Geometry check sheet. Reference: drawing and pictorial views, mm from the part's lowest x, y, z. Coordinates: 2 decimals unless noted, no trailing zeros. Loops run counter-clockwise (first coordinate to the right, second up) from the corner with the lowest first, then second, coordinate; pieces in that order, holes last. Notation, with made-up numbers: (75.5, -27) -> (80.5, -27) arc R30 cw to (80.5, -4) -> close; hole circle Ø8 at (83, 40). An arc over 180 degrees is marked (long way). Answer as a JSON object with one key per item and string values.
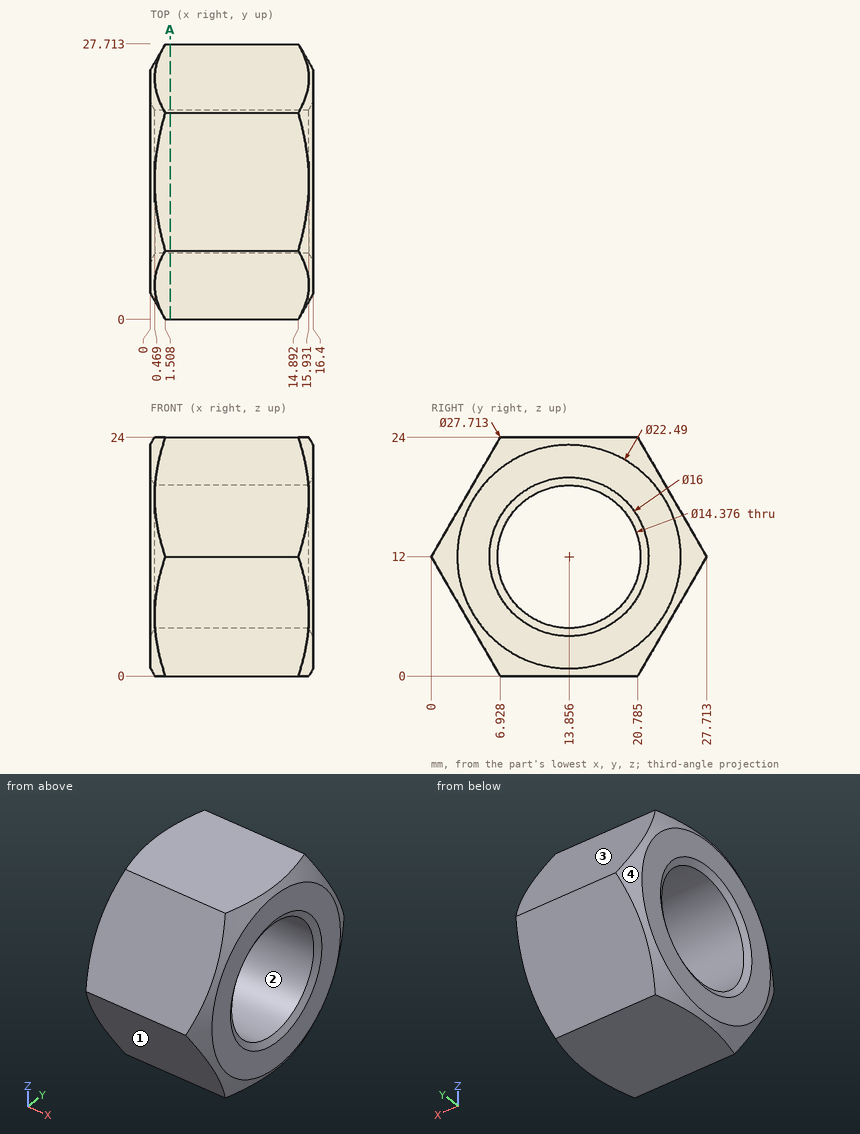
1. Section check A-A, the plane x = 2. Record the boundary of the cut face in (y, z) (1 decimal).
Evaluation:
{"outline": "(0, 12) -> (6.9, 0) -> (20.8, 0) -> (27.7, 12) -> (20.8, 24) -> (6.9, 24) -> close; hole circle Ø14.4 at (13.9, 12)"}
2. Thickness scan on probe 1 along Z at (x, y) = (3, 9); probe 2 along Y at (x, z) = (1.5, 7) (1 decimal); probe 3 along Y at (x, z) = (6, 6.5) (1 decimal). Record the ranges inside material, lowest first. Write a range as from..to.
Evaluation:
{"probe 1": "z = 0..6.7, 17.3..24", "probe 2": "y = 2.9..8.7, 19..24.8", "probe 3": "y = 3.2..9.2, 18.5..24.5"}
3. Mould release check, pull along Z, two halves, no side actions. Record for the marked faces 1, 2, 3 and 4: released by +Z, released by -Z, zero draft, split by the parting line, or undercut.
Evaluation:
{"face 1": "released by -Z", "face 2": "undercut", "face 3": "released by +Z", "face 4": "split by the parting line"}
4. Depth check by flat-ended pin: P1, Ø3, axis at x = 14, z = 5, coming from the +Y side; P2, Ø1.5, axis at x = 8.5, y = 24, coming from the -Z side; P3, Ø1, axis at y = 19, z = 13.5, coming from the +X side. Enter the tip coordinate at first touch or a pass-through.
Evaluation:
{"P1": "stops at y = 24.54", "P2": "stops at z = 4.27", "P3": "passes through"}
